from build123d import *

# Parameters (mm, degrees)
F3_D     = 45
F3_DEPTH = 20
F3_TIP   = 13.5193639281
F5_D     = 3.3
F5_DEPTH = 20
F5_TIP   = 0.9914200214


with BuildPart() as f1:
    # F0 (on Right) → F1 (revolve)
    with BuildSketch(Plane.YZ):
        Polygon((0, -2.6000006461), (0, 0), (-26, 0), (-26, -25), (-33.4, -25), (-33.4, -27.5), (-23.4, -27.5), (-23.4, -24.5), (-21.4, -24.5), (-21.4, -20), (-23.4, -20), (-23.4, -2.6000006461), align=None)
    revolve(axis=Axis((0, 0, -1.300000323), (0, 0, 1)))

    # F3
    with Locations(Plane.XY):
        with Locations((0, 0)):
            Hole(F3_D / 2, depth=F3_DEPTH)
            with Locations((0, 0, -(F3_DEPTH + F3_TIP / 2))):  # 118° drill point
                Cone(0, F3_D / 2, F3_TIP, mode=Mode.SUBTRACT)

    # F5
    with Locations(Plane.XY.offset(-25)):
        with Locations((-26.1672226652, 13.4486109676), (-17.3401695769, 23.7677764633), (-5.3680126756, 28.9270309378), (9.997338267, 27.6702350286), (21.5074325556, 20.0753337165), (27.2051514467, 11.2012683982), (29.4208884802, 0), (27.6971504759, -9.9225266177), (23.0558330823, -18.2761385376), (15.1375992814, -25.2277975051), (4.1127317731, -29.1320118826), (-8.323613721, -28.2188967465), (-17.0114493372, -24.0041511079), (-23.7931689823, -17.3053109983), (-29.4208884802, 0), (-27.5693241627, -10.2723436556)):
            Hole(F5_D / 2, depth=F5_DEPTH)
            with Locations((0, 0, -(F5_DEPTH + F5_TIP / 2))):  # 118° drill point
                Cone(0, F5_D / 2, F5_TIP, mode=Mode.SUBTRACT)


solid = f1.part
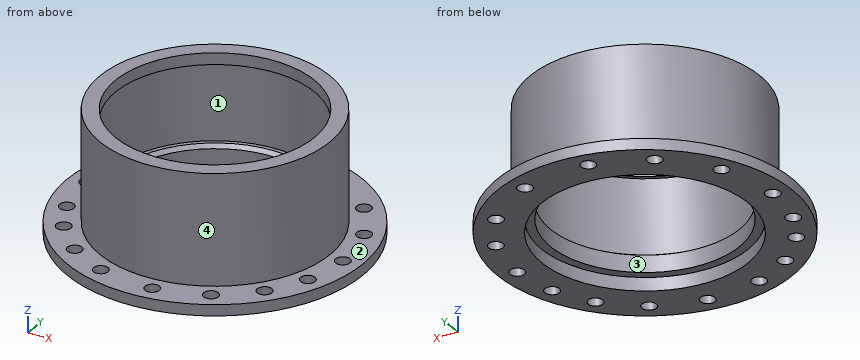
Read the model definition and answer for the solid it produces. Units are mm, in the model's axes. Face numbers are marked on the shaded views. Coordinates: 2 decimals unless noted, no trailing zeros. Order: outer loops, then holes, each group sorted by start corner. A loop starts at its lowest first (then second) coordinate and runs counter-clockwise, first axis right, second up. Notation, with made-up numbers: (-7, 69) -> (4, 69) arc R18 cw to (4, 86) -> close; hole circle Ø2 at (53, 75). An arc over 180 degrees is marked (long way). Answer as a JSON object with one key per item and string values.
1) A cutting plane is placed at C-C, the plane z = -14. Determine the outline of the cut face in (x, y).
Model answer:
{"outline": "circle Ø52 at (0, 0); hole circle Ø46.8 at (0, 0)"}
2) Each of these flat-tipped pins is pushed along its axis until it touches: pin 1 (4 mm diameter, centred on x = -10, y = 17, fed in from -Z); pin 2 (2.5 mm diameter, centred on x = 4.11, y = -29.13, fed in from -Z); pin 3 (8 mm diameter, centred on y = -26.5, z = -3, fed in from -X); pin 4 (10 mm diameter, centred on x = 7, z = -24, fed in from -Y). Where does it stop, or does it pass through?
Model answer:
{"pin 1": "stops at z = -24.5", "pin 2": "passes through", "pin 3": "stops at x = -13.03", "pin 4": "stops at y = -33.33"}
3) The mould has two halves that part along Y. Classify the marked faces 1, 2, 3 and 4: released by +Y, released by -Y, zero draft, split by the parting line, or undercut.
Model answer:
{"face 1": "undercut", "face 2": "zero draft", "face 3": "undercut", "face 4": "split by the parting line"}
4) Consider line 1 along X through (y, z) = (0, -14); line 2 along Z through (x, y) = (-8.5, -21); line 3 along Y through (x, z) = (16, -19). Determine where each line is inside the solid, lowest interval first. Write a range as from..to.
Model answer:
{"line 1": "x = -26..-23.4, 23.4..26", "line 2": "z = -24.5..-20, -2.6..0", "line 3": "y = -20.49..-17.08, 17.08..20.49"}
5) A cutting plane is placed at D-D, the plane z = -21.75. Determine the outline of the cut face in (x, y).
Model answer:
{"outline": "circle Ø52 at (0, 0); hole circle Ø42.8 at (0, 0)"}
6) A cutting plane is placed at A-A, the plane y = 0. State how many separate pieces and enclosed holes the cut face has, plus the area to 3 significant figures.
Model answer:
{"separate pieces": "4", "enclosed holes": "0", "area": "185 mm²"}
7) A cutting plane is placed at B-B, the plane x = 0. Determine the outline of the cut face in (y, z), plus the area to 3 significant figures.
Model answer:
{"outline": "(-33.4, -27.5) -> (-23.4, -27.5) -> (-23.4, -24.5) -> (-21.4, -24.5) -> (-21.4, -20.66) -> (-22.5, -20) -> (-23.4, -20) -> (-23.4, -2.6) -> (-22.5, -2.6) -> (-22.5, 0) -> (-26, 0) -> (-26, -25) -> (-33.4, -25) -> close; (21.4, -24.5) -> (23.4, -24.5) -> (23.4, -27.5) -> (33.4, -27.5) -> (33.4, -25) -> (26, -25) -> (26, 0) -> (22.5, 0) -> (22.5, -2.6) -> (23.4, -2.6) -> (23.4, -20) -> (22.5, -20) -> (21.4, -20.66) -> close", "area": "202 mm²"}
